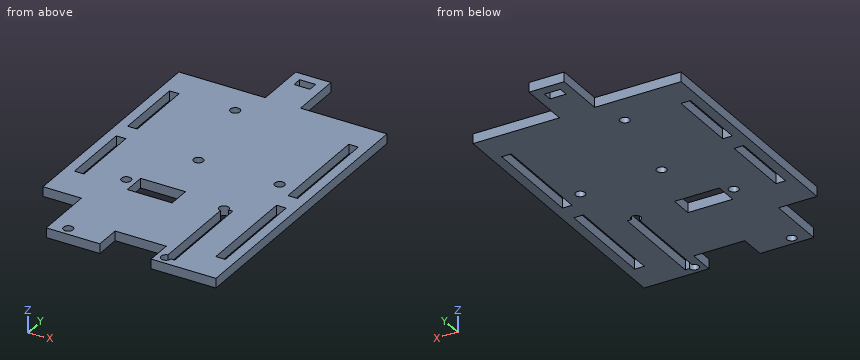
from build123d import *

# Parameters (mm, degrees)
SKETCH1_W           = 65
SKETCH1_H           = 90
BOSS_EXTRUDE1_DEPTH = 3
SKETCH3_R           = 1.5
CUT_EXTRUDE2_DEPTH  = 3
SKETCH4_R           = 1.5
CUT_EXTRUDE3_DEPTH  = 4
SKETCH5_W           = 3
SKETCH5_H           = 32
CUT_EXTRUDE4_DEPTH  = 4
SKETCH6_W           = 3
SKETCH6_H           = 22
CUT_EXTRUDE5_DEPTH  = 4
SKETCH7_W           = 3
SKETCH7_H           = 30.5
SKETCH7_W_2         = 14
SKETCH7_H_2         = 7
SKETCH7_W_3         = 16
SKETCH7_H_3         = 8
CUT_EXTRUDE6_DEPTH  = 4
SKETCH8_W           = 12
SKETCH8_H           = 18.5
CUT_EXTRUDE7_DEPTH  = 4
SKETCH10_W          = 11
SKETCH10_H          = 16
SKETCH10_W_2        = 5
SKETCH10_H_2        = 3
BOSS_EXTRUDE3_DEPTH = 3


with BuildPart() as part:
    # Sketch1 → Boss-Extrude1 (new body)
    with BuildSketch(Plane.XY):
        Rectangle(SKETCH1_W, SKETCH1_H)
    extrude(amount=-BOSS_EXTRUDE1_DEPTH)

    # Sketch3 → Cut-Extrude2 (cut)
    with BuildSketch(Plane.XY):
        with Locations((-8.98, 35)):
            Circle(SKETCH3_R)
        with Locations((-3.9, 7.06)):
            Circle(SKETCH3_R)
        with Locations((21.5, 7.06)):
            Circle(SKETCH3_R)
    extrude(amount=-CUT_EXTRUDE2_DEPTH, mode=Mode.SUBTRACT)

    # Sketch4 → Cut-Extrude3 (cut, through all)
    with BuildSketch(Plane.XY):
        with Locations((-15.25, -42.25)):
            Circle(SKETCH4_R)
        with Locations((-15.25, -11.75)):
            Circle(SKETCH4_R)
        with Locations((15.25, -42.25)):
            Circle(SKETCH4_R)
        with Locations((15.25, -11.75)):
            Circle(SKETCH4_R)
    extrude(amount=-CUT_EXTRUDE3_DEPTH, mode=Mode.SUBTRACT)

    # Sketch5 → Cut-Extrude4 (cut, through all)
    with BuildSketch(Plane.XY):
        with Locations((28, -19)):
            Rectangle(SKETCH5_W, SKETCH5_H)
        with Locations((28, 19)):
            Rectangle(SKETCH5_W, SKETCH5_H)
    extrude(amount=-CUT_EXTRUDE4_DEPTH, mode=Mode.SUBTRACT)

    # Sketch6 → Cut-Extrude5 (cut, through all)
    with BuildSketch(Plane.XY):
        with Locations((-28, -4)):
            Rectangle(SKETCH6_W, SKETCH6_H)
        with Locations((-28, 24)):
            Rectangle(SKETCH6_W, SKETCH6_H)
    extrude(amount=-CUT_EXTRUDE5_DEPTH, mode=Mode.SUBTRACT)

    # Sketch7 → Cut-Extrude6 (cut, through all)
    with BuildSketch(Plane.XY):
        with Locations((16.5, -27)):
            Rectangle(SKETCH7_W, SKETCH7_H)
        with Locations((-5.25, -12.75)):
            Rectangle(SKETCH7_W_2, SKETCH7_H_2)
        with Locations((4.25, -41)):
            Rectangle(SKETCH7_W_3, SKETCH7_H_3)
    extrude(amount=-CUT_EXTRUDE6_DEPTH, mode=Mode.SUBTRACT)

    # Sketch8 → Cut-Extrude7 (cut, through all)
    with BuildSketch(Plane.XY):
        with Locations((-26.5, -35.75)):
            Rectangle(SKETCH8_W, SKETCH8_H)
    extrude(amount=-CUT_EXTRUDE7_DEPTH, mode=Mode.SUBTRACT)

    # Sketch10 → Boss-Extrude3 (add)
    with BuildSketch(Plane.XY):
        with Locations((0, 53)):
            Rectangle(SKETCH10_W, SKETCH10_H)
        with Locations((0, 56.5)):
            Rectangle(SKETCH10_W_2, SKETCH10_H_2, mode=Mode.SUBTRACT)
    extrude(amount=-BOSS_EXTRUDE3_DEPTH)


solid = part.part
The model under review builds one solid part; all positions refer to its coordinate system, in mm. Give positions to 0.01 mm unless a question says otherwise; leave off trailing zeros. Order: outer loops, then holes, each group sorted by start corner. A loop starts at its lowest first (then second) coordinate and runs counter-clockwise, first axis right, second up. Notation, with made-up numbers: M 2,14 L 20,14 A38 ccw 20,53 Z; hole C 68.5,86.25 d9. An arc over 180 degrees is marked long. Use one line per item in the form item = value. Start each with the question number.
Item 1: We need section B-B on y = -36. Give the boundary of the cut face in (x, z), plus the area to 3 significant figures.
Item 2: We need section A-A on x = -8.98. Give the boundary of the cut face in (y, z).
Item 3: We need section C-C on x = 21.5. Give the boundary of the cut face in (y, z), plus the area to 3 significant figures.
Item 4: Insertion check: pin 1 Ø3 at (x, y) = (-1.5, 39.5) entering from +Z; pin 2 Ø0.9 at (x, z) = (-2, -1) entering from -Y; pin 3 Ø0.9 at (x, z) = (27.5, -1) entering from +Y. Each pin has a flat end and moves straight along its axis. Give the tip position at first contact, or say it passes through.
Item 5: We need section D-D on z = -1.4. Give the number of separate pieces and of enclosed holes in the cut face, plus the area to 3 significant figures.
Item 6: To check wall thickness, follow line 1 along Y through (x, z) = (-15.25, -1.9); line 2 along X through (y, z) = (14.5, -0.6); line 3 along X through (y, z) = (-20, -0.9). State the ranges of each line that lie inside material, in increasing order. Write a range as from..to.
Completed:
q1.outline = M -20.5,-3 L 15,-3 L 15,0 L -20.5,0 Z; M 18,-3 L 32.5,-3 L 32.5,0 L 18,0 Z
q1.area = 150 mm²
q2.outline = M -45,-3 L -16.25,-3 L -16.25,0 L -45,0 Z; M -9.25,-3 L 33.5,-3 L 33.5,0 L -9.25,0 Z; M 36.5,-3 L 45,-3 L 45,0 L 36.5,0 Z
q3.outline = M -45,-3 L 5.56,-3 L 5.56,0 L -45,0 Z; M 8.56,-3 L 45,-3 L 45,0 L 8.56,0 Z
q3.area = 261 mm²
q4.pin_1 = 0
q4.pin_2 = -37
q4.pin_3 = 45
q5.separate_pieces = 1
q5.enclosed_holes = 12
q5.area = 5,100 mm²
q6.line_1 = -45..-43.75, -40.75..-13.25, -10.25..45
q6.line_2 = -32.5..-29.5, -26.5..26.5, 29.5..32.5
q6.line_3 = -32.5..15, 18..26.5, 29.5..32.5
